Could you check a few things on this model? Use its own coordinates, in mm. A direction names the side the tool comes from. Coordinates: 2 decimals unless noted, no trailing zeros. Order: outer loops, then holes, each group sorted by start corner. A loop starts at its lowest first (then second) coordinate and runs counter-clockwise, first axis right, second up. Notation, with made-up numbers: (-9, 58) -> (5, 58) arc R12 ccw to (5, 79) -> close; hole circle Ø8 at (-27, 42.5). An arc over 180 degrees is marked (long way). Put each result on its own line as item: value. Start each with the question number.
Q1. For faces 1 (the face through (-47, 44.45, 3)), 2 (the face through (19.05, 63, 3)), 3 (the face through (-32.568, -42.713, 3.219)), which set-ups out of +Z, -Z, +X, -X, +Y, -Y let a thin tool reach every point of the face, with its end or its side?
Q2. If we section it at D-D (x = -22): Please give me the cut outline in (y, z) (3 decimals).
Q3. If we section it at B-B (x = -44.45): Please give me the cut outline in (y, z).
Q4. If we section it at C-C (z = 2.5): Count the separate pieces of the cut face and the enclosed holes in it, and give its area (3 significant figures).
Q5. Please list where these lines run through material, in increasing order: line 1 along Y through (x, z) = (-44.45, 5); line 2 along X through (y, z) = (-37.5, 2.75); line 3 along Y through (x, z) = (0, 2.5).
Q6. If we section it at A-A (y = -25.4): Please give me the cut outline in (x, z).
Q7. We'd pull the mould along X, two halves only. Please class faces 4 (the face through (-19.17, -25.58, 3.13)), 5 (the face through (-63.5, 8, 3)), 6 (the face through (-3.103, 49.527, 3.219)): +X half, -X half, draft (parallel to the pull), parting line (faces both ways), or undercut.
Q8. Will these pins go through, and if not, where does the flat tip stop? pin 1 (17 mm diameter, centred on x = 0, y = 63.5, fed in from +Z); pin 2 (1.9 mm diameter, centred on y = 62.5, z = 4.5, fed in from +X); pin 3 (3 mm diameter, centred on x = -3.5, y = 4.5, fed in from -Z); pin 4 (3 mm diameter, centred on x = 42.5, z = 2, fed in from +Y).
from build123d import *

# Parameters (mm, degrees)
SKETCH1_R           = 14.3129
BOSS_EXTRUDE1_DEPTH = 6.35
FILLET1_R           = 14.2875
SKETCH2_W           = 38.1
SKETCH2_H           = 38.1
BOSS_EXTRUDE2_DEPTH = 6.35
FILLET2_R           = 14.2875
SKETCH3_R           = 14.3129
CUT_EXTRUDE1_DEPTH  = 105.341147205
FILLET3_R           = 12.7


with BuildPart() as part:
    # Sketch1 → Boss-Extrude1 (new body)
    with BuildSketch(Plane.XY):
        Polygon((-6.35, -6.35), (63.5, -6.35), (63.5, 44.45), (-63.5, 44.45), (-63.5, -44.45), (-31.75, -44.45), align=None)
        with Locations((-44.45, -25.4)):
            Circle(SKETCH1_R, mode=Mode.SUBTRACT)
        with Locations((35.871852568, 12.7)):
            Circle(SKETCH1_R, mode=Mode.SUBTRACT)
    extrude(amount=BOSS_EXTRUDE1_DEPTH)

    # Fillet1
    fillet1_edges = [part.edges().sort_by_distance(p)[0] for p in [
        (-31.75, -44.45, 3.175),
        (-63.5, -44.45, 3.175),
        (63.5, -6.35, 3.175),
        (-6.35, -6.35, 3.175),
    ]]
    fillet(fillet1_edges, radius=FILLET1_R)

    # Sketch2 → Boss-Extrude2 (add)
    with BuildSketch(Plane.XY.offset(6.35)):
        with Locations((0, 63.5)):
            Rectangle(SKETCH2_W, SKETCH2_H)
    extrude(amount=-BOSS_EXTRUDE2_DEPTH)

    # Fillet2
    fillet2_edges = [part.edges().sort_by_distance(p)[0] for p in [
        (-19.05, 82.55, 3.175),
        (19.05, 82.55, 3.175),
        (19.05, 44.45, 3.175),
    ]]
    fillet(fillet2_edges, radius=FILLET2_R)

    # Sketch3 → Cut-Extrude1 (cut, through all)
    with BuildSketch(Plane.XY.offset(6.35)):
        with Locations((0, 63.5)):
            Circle(SKETCH3_R)
    extrude(amount=-CUT_EXTRUDE1_DEPTH, mode=Mode.SUBTRACT)

    # Fillet3
    fillet3_edges = [part.edges().sort_by_distance(p)[0] for p in [
        (-19.05, 44.45, 3.175),
    ]]
    fillet(fillet3_edges, radius=FILLET3_R)


solid = part.part
The answers:
1. face 1: +Z, -Z, -X, +Y
1. face 2: +Z, -Z, +X, +Y
1. face 3: +Z, -Z, +X, -Y
2. outline: (-29.825, 0) -> (49.012, 0) -> (49.012, 6.35) -> (-29.825, 6.35) -> close
3. outline: (-44.45, 0) -> (-39.71, 0) -> (-39.71, 6.35) -> (-44.45, 6.35) -> close; (-11.09, 0) -> (44.45, 0) -> (44.45, 6.35) -> (-11.09, 6.35) -> close
4. separate pieces: 1
4. enclosed holes: 3
4. area: 7,570 mm^2
5. line 1: -44.45 to -39.71, -11.09 to 44.45
5. line 2: -61.47 to -52.1, -36.8 to -27.12
5. line 3: -6.41 to 49.19, 77.81 to 82.55
6. outline: (-63.5, 0) -> (-58.76, 0) -> (-58.76, 6.35) -> (-63.5, 6.35) -> close; (-30.14, 0) -> (-19.05, 0) -> (-19.05, 6.35) -> (-30.14, 6.35) -> close
7. face 4: +X half
7. face 5: -X half
7. face 6: undercut
8. pin 1: through
8. pin 2: x = 19.05
8. pin 3: z = 0
8. pin 4: y = 44.45
